Answer from the drawing. Dimensions are ordinates in mm from the lowest x, y and z of the part. A direction names the side the tool comes from. Coordinates: 2 decimals unless noted, no trailing zeros. Order: outer loops, then holes, each group sorted by start corner. A loop starts at its lowest first (then second) coordinate and runs counter-clockwise, first axis right, second up. Notation, with made-up numbers: (49, -35) - (96, -35) arc R26 ccw to (96, -17) - close; hole circle Ø8 at (39, -32). An arc over 180 degrees is marked (long way). Answer as a JSON object with one key per item and string values. Group by question number.
1) Section B-B (y = 40) is taken. Give the vertices of the cut face in (x, z).
2) Section C-C (z = 65) is taken. Give the vertices of the cut face in (x, y), plus the area to 3 significant figures.
3) Find the intervals of material crossed by line 1 along X through (y, z) = (72, 65); line 2 along Y through (x, z) = (42, 30.5); line 3 along Z through (x, y) = (15, 21.5), in increasing order.
4) The mould has two halves that part along Y. Classify the marked faces 3, 4 and 5: released by +Y, released by -Y, zero draft, split by the parting line, or undercut.
5) A tool of negligible diameter and unlimited length cuts with its end or side. For the marked faces 1 and 2, from which of +Z, -Z, +X, -X, +Y, -Y can it reach the whole face along a straight path? Write none if from no direction.
6) Section D-D (z = 82) is taken. Give the vertices of the cut face in (x, y).
7) Section A-A (x = 40) is taken. Give the vertices of the cut face in (y, z).
8) Each of these flat-tipped pins is pushed along its axis until it touches: P1, Ø9.5, axis at x = 40, y = 40, coming from the +Z side; P2, Ø3.5, axis at x = 40, z = 65, coming from the -Y side. Where does it stop, or does it pass through?
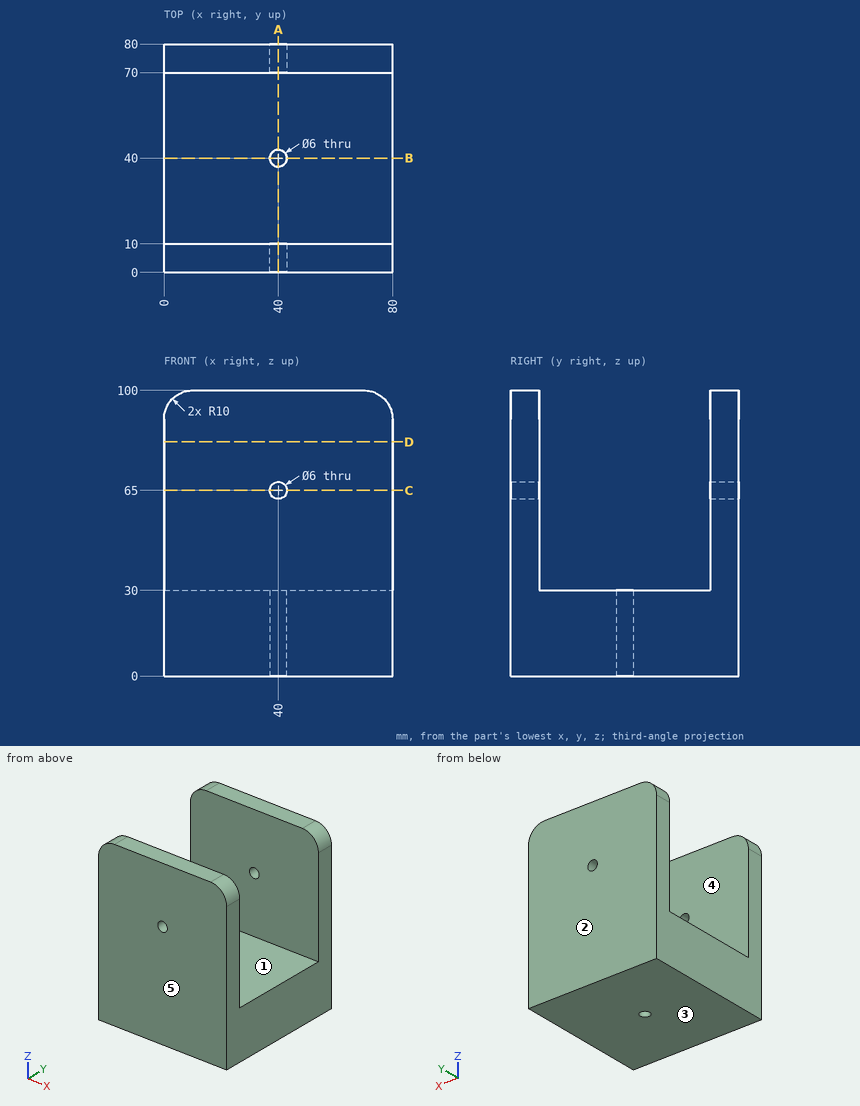
Report:
{
 "1": {"outline": "(0, 0) - (37, 0) - (37, 30) - (0, 30) - close; (43, 0) - (80, 0) - (80, 30) - (43, 30) - close"},
 "2": {"outline": "(0, 0) - (37, 0) - (37, 10) - (0, 10) - close; (0, 70) - (37, 70) - (37, 80) - (0, 80) - close; (43, 0) - (80, 0) - (80, 10) - (43, 10) - close; (43, 70) - (80, 70) - (80, 80) - (43, 80) - close", "area": "1,480 mm²"},
 "3": {"line 1": "x = 0 to 37, 43 to 80", "line 2": "y = 0 to 10, 70 to 80", "line 3": "z = 0 to 30"},
 "4": {"face 3": "zero draft", "face 4": "undercut", "face 5": "released by -Y"},
 "5": {"face 1": "+Z, +X, -X", "face 2": "+Z, -Z, +X, -X, +Y"},
 "6": {"outline": "(0, 0) - (80, 0) - (80, 10) - (0, 10) - close; (0, 70) - (80, 70) - (80, 80) - (0, 80) - close"},
 "7": {"outline": "(0, 0) - (37, 0) - (37, 30) - (10, 30) - (10, 62) - (0, 62) - close; (0, 68) - (10, 68) - (10, 100) - (0, 100) - close; (43, 0) - (80, 0) - (80, 62) - (70, 62) - (70, 30) - (43, 30) - close; (70, 68) - (80, 68) - (80, 100) - (70, 100) - close"},
 "8": {"P1": "stops at z = 30", "P2": "passes through"}
}
